Here's how the part is built. I have some questions about the finished solid (model axes, mm). A direction names the side the tool comes from. Round coordinates to 2 decimals unless told otherwise and drop trailing zeros. Order: outer loops, then holes, each group sorted by start corner. A loop starts at its lowest first (then second) coordinate and runs counter-clockwise, first axis right, second up.
```python
from build123d import *

# Parameters (mm, degrees)
F0_W     = 104.775
F0_H     = 68.2625
F1_DEPTH = 4.7625
F2_W     = 2.38125
F2_H     = 2.38125
F3_DEPTH = 104.775
F4_R     = 1.5875
F5_DEPTH = 4.7625


with BuildPart() as f1:
    # F0 (on Front) → F1 (new body)
    with BuildSketch(Plane.XZ):
        Rectangle(F0_W, F0_H)
    extrude(amount=F1_DEPTH)

    # F2 (on face) → F3 (cut, through all)
    with BuildSketch(Plane.YZ.offset(52.3875)):
        with Locations((-3.571875, 32.940625)):
            Rectangle(F2_W, F2_H)
        with Locations((-3.571875, -32.940625)):
            Rectangle(F2_W, F2_H)
    extrude(amount=-F3_DEPTH, mode=Mode.SUBTRACT)

    # F4 (on face) → F5 (cut, through all)
    with BuildSketch(Plane.XZ.offset(4.7625)):
        with Locations((-49.2125, 28.575)):
            Circle(F4_R)
        with Locations((49.2125, 28.575)):
            Circle(F4_R)
        with Locations((-49.2125, -28.575)):
            Circle(F4_R)
        with Locations((49.2125, -28.575)):
            Circle(F4_R)
    extrude(amount=-F5_DEPTH, mode=Mode.SUBTRACT)


solid = f1.part
```
1. If we mould it in two halves opening along X, with no side actions, what happens to faces 1 (the cylindrical face through (50.07, -2.41, -27.24)), 2 (the flat face through (-52.388, -2, 0)), 3 (the flat face through (1, -4, -31.75)), 4 (the cylindrical face through (-48.359, -2.415, -27.236))? For each: released by +X, released by -X, zero draft, split by the parting line, or undercut.
Evaluation:
face 1: undercut
face 2: released by -X
face 3: zero draft
face 4: undercut
2. I need wall thicknesses on probe 1 along Z at (x, y) = (-33, -4). Which ranges of the line are inside material? Lowest first, please.
Evaluation:
probe 1: z = -31.75 to 31.75
3. If we section it at A-A, the plane x = 0.5: Write out the boundary of the cut face in (y, z), and give its area (3 significant figures).
Evaluation:
outline: (-4.76, -31.75) - (-2.38, -31.75) - (-2.38, -34.13) - (0, -34.13) - (0, 34.13) - (-2.38, 34.13) - (-2.38, 31.75) - (-4.76, 31.75) - close
area: 314 mm2
4. I'm going to push flat-ended pins straight in: P1, Ø2.5, axis at x = -5, z = -32.5, coming from the -Y side; P2, Ø2, axis at x = -21, y = -4, coming from the +Z side. Where does each tip first touch, or does it pass through?
Evaluation:
P1: stops at y = -4.76
P2: stops at z = 31.75
5. On a 3-axis mill with a long thin cutter (end or side, diameter ignored), from which of +Z, -Z, +X, -X, +Y, -Y can I reach the whole of each face in a straight line? I mean faces 5 (the cylindrical face through (49, -2, 27)), 6 (the flat face through (1, -2.381, 33)), 7 (the flat face through (1, -2.381, -33)). Say none if no direction works.
Evaluation:
face 5: +Y, -Y
face 6: +Z, +X, -X, -Y
face 7: -Z, +X, -X, -Y
6. If we section it at B-B, the plane y = -4: State how many separate pieces and enclosed holes the cut face has, and give its area (3 significant figures).
Evaluation:
separate pieces: 1
enclosed holes: 4
area: 6,620 mm2
